Part model, mm, in its own coordinate system. Face numbers are marked on the shaded views. A direction names the side the tool comes from. Round coordinates to 2 decimals unless told otherwise and drop trailing zeros. Write each loop counter-clockwise with the first axis right and the second up, starting at its lowest first coordinate (ties: lowest second). Pieces come first, ordered by that corner, then holes.
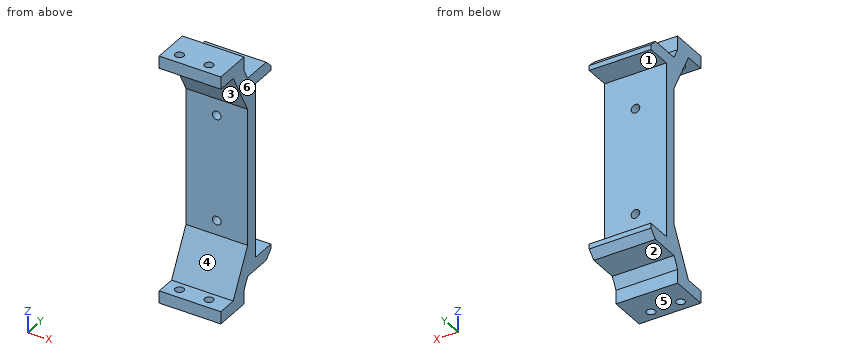
from build123d import *

# Parameters (mm, degrees)
CYLINDER024_R          = 1.75
CYLINDER024_DEPTH      = 20
CYLINDER023_R          = 1.75
CYLINDER023_DEPTH      = 20
CYLINDER022_R          = 1.75
CYLINDER022_DEPTH      = 20
CYLINDER021_R          = 1.75
CYLINDER021_DEPTH      = 20
CYLINDER018_R          = 1.75
CYLINDER018_DEPTH      = 20
CYLINDER018_ROLL_ANGLE = 90
CYLINDER017_R          = 1.75
CYLINDER017_DEPTH      = 20
CYLINDER017_ROLL_ANGLE = 90
PAD006_DEPTH           = 25
CHAMFER006_SIZE        = 3


with BuildPart() as cylinder059:
    # Cylinder024 → Cylinder024 (new body)
    with BuildSketch(Plane(origin=(40, -18, -24), x_dir=(1, 0, 0), z_dir=(0, 0, 1))):
        Circle(CYLINDER024_R)
    extrude(amount=CYLINDER024_DEPTH)


with BuildPart() as cylinder058:
    # Cylinder023 → Cylinder023 (new body)
    with BuildSketch(Plane(origin=(28, -18, -24), x_dir=(1, 0, 0), z_dir=(0, 0, 1))):
        Circle(CYLINDER023_R)
    extrude(amount=CYLINDER023_DEPTH)


with BuildPart() as cylinder057:
    # Cylinder022 → Cylinder022 (new body)
    with BuildSketch(Plane(origin=(40, -18, 77), x_dir=(1, 0, 0), z_dir=(0, 0, 1))):
        Circle(CYLINDER022_R)
    extrude(amount=CYLINDER022_DEPTH)


with BuildPart() as cylinder056:
    # Cylinder021 → Cylinder021 (new body)
    with BuildSketch(Plane(origin=(28, -18, 77), x_dir=(1, 0, 0), z_dir=(0, 0, 1))):
        Circle(CYLINDER021_R)
    extrude(amount=CYLINDER021_DEPTH)


with BuildPart() as cylinder053:
    # Cylinder018 → Cylinder018 (new body)
    with BuildSketch(Plane.XY):
        Circle(CYLINDER018_R)
    extrude(amount=CYLINDER018_DEPTH)


with BuildPart() as cylinder053_1:
    # Cylinder018 roll: moved
    add(cylinder053.part.rotate(Axis((0, 0, 0), (1, 0, 0)), CYLINDER018_ROLL_ANGLE))


with BuildPart() as cylinder053_2:
    # Cylinder018 placement: moved
    add(cylinder053_1.part.moved(Location((35, 10, 13))))


with BuildPart() as cylinder052:
    # Cylinder017 → Cylinder017 (new body)
    with BuildSketch(Plane.XY):
        Circle(CYLINDER017_R)
    extrude(amount=CYLINDER017_DEPTH)


with BuildPart() as cylinder052_1:
    # Cylinder017 roll: moved
    add(cylinder052.part.rotate(Axis((0, 0, 0), (1, 0, 0)), CYLINDER017_ROLL_ANGLE))


with BuildPart() as cylinder052_2:
    # Cylinder017 placement: moved
    add(cylinder052_1.part.moved(Location((35, 10, 56))))


with BuildPart() as obj1:
    # Sketch012 → Pad006 (new body)
    with BuildSketch(Plane(origin=(47.5, 0, -0.5), x_dir=(0, 0, 1), z_dir=(-1, 0, 0))):
        Polygon((-0.046577, 10.001707), (-0.046577, 0.001707), (70.953423, 0.001707), (70.953423, 10.001707), (75.953423, 10.001707), (75.953423, -4.998293), (80.375589, -7.331627), (85.953423, -7.331627), (85.953423, -22.331627), (80.953423, -22.331627), (80.953423, -14.331627), (63.264757, -4.998293), (7.642088, -4.998293), (-10.046577, -14.331627), (-10.046577, -22.331627), (-15.046577, -22.331627), (-15.046577, -7.331627), (-9.468744, -7.331627), (-5.046577, -4.998293), (-5.046577, 10.001707), align=None)
    extrude(amount=PAD006_DEPTH)

    # Cut037: cut Cylinder052
    add(cylinder052_2.part, mode=Mode.SUBTRACT)

    # Cut038: cut Cylinder053
    add(cylinder053_2.part, mode=Mode.SUBTRACT)

    # Cut045: cut Cylinder056
    add(cylinder056.part, mode=Mode.SUBTRACT)

    # Cut046: cut Cylinder057
    add(cylinder057.part, mode=Mode.SUBTRACT)

    # Cut047: cut Cylinder058
    add(cylinder058.part, mode=Mode.SUBTRACT)

    # Cut048: cut Cylinder059
    add(cylinder059.part, mode=Mode.SUBTRACT)

    # Chamfer006
    chamfer006_edges = [obj1.edges().sort_by_distance(p)[0] for p in [
        (35, 10.001707, 75.453423),
        (35, 10.001707, -5.546577),
    ]]
    chamfer(chamfer006_edges, length=CHAMFER006_SIZE)


solid = obj1.part
Q1. Saw through at A-A, the plane y = -18. Write the cut outline in (x, z), and give its area (3 significant figures).
Q2. Saw through at D-D, the plane y = -1. Write the cut outline in (x, z), and give its area (3 significant figures).
Q3. Two-plate mould, pull along Z, no slides. Class the marked faces 4, 5 and 6: released by +Z, released by -Z, zero draft, split by the parting line, or undercut.
Q4. Drop flat-ended pins along their axis: P1, Ø7.5, axis at x = 29, z = 29, coming from the +Y side; P2, Ø8, axis at x = 33, y = 3.5, coming from the +Z side; P3, Ø5, axis at x = 37, y = 7, coming from the -Z side. Give the stop position or say it passes through.
Q5. Saw through at B-B, the plane x = 28.75. Give the number of separate pieces and of enclosed holes in the cut face, and give its area (3 significant figures).
Q6. Tool access for the marked faces 1, 2 and 3: list every direction of +Z, -Z, +X, -X, +Y, -Y with a clear straight run to the whole face (end or side of a thin tool).
Q7. Wall check: line 1 (Z direction, x = 35, y = -1.25); line 2 (X direction, y = -18, z = 83); line 3 (Y direction, x = 28, z = 82.9). Give the ranges that are in metal, low to high.
Q8. Saw through at C-C, the plane y = 5. Write the cut outline in (x, z).
Computed:
1. outline: (22.5, -15.55) - (26.25, -15.55) - (26.25, -10.55) - (22.5, -10.55) - close; (22.5, 80.45) - (26.25, 80.45) - (26.25, 85.45) - (22.5, 85.45) - close; (29.75, -15.55) - (38.25, -15.55) - (38.25, -10.55) - (29.75, -10.55) - close; (29.75, 80.45) - (38.25, 80.45) - (38.25, 85.45) - (29.75, 85.45) - close; (41.75, -15.55) - (47.5, -15.55) - (47.5, -10.55) - (41.75, -10.55) - close; (41.75, 80.45) - (47.5, 80.45) - (47.5, 85.45) - (41.75, 85.45) - close
1. area: 180 mm2
2. outline: (22.5, -5.55) - (47.5, -5.55) - (47.5, 75.45) - (22.5, 75.45) - close; hole circle Ø3.5 at (35, 13); hole circle Ø3.5 at (35, 56)
2. area: 2,010 mm2
3. face 4: undercut
3. face 5: released by -Z
3. face 6: zero draft
4. P1: stops at y = 0
4. P2: stops at z = 75.45
4. P3: stops at z = -5.55
5. separate pieces: 3
5. enclosed holes: 0
5. area: 766 mm2
6. face 1: +X, -X, +Y
6. face 2: -Z, +X, -X, +Y
6. face 3: +X, -X, -Y
7. line 1: z = -5.55 to 11.25, 14.75 to 54.25, 57.75 to 75.45
7. line 2: x = 22.5 to 26.25, 29.75 to 38.25, 41.75 to 47.5
7. line 3: y = -22.33 to -19.75, -16.25 to -7.33
8. outline: (22.5, -5.55) - (47.5, -5.55) - (47.5, -0.55) - (22.5, -0.55) - close; (22.5, 70.45) - (47.5, 70.45) - (47.5, 75.45) - (22.5, 75.45) - close
